```python
from build123d import *

# Parameters (mm, degrees)
BOSS_EXTRUDE1_DEPTH = 3.175
FILLET1_R           = 0.5
CUT_EXTRUDE2_REACH  = 51.643
SKETCH3_R           = 0.9652
FILLET2_R           = 1.5


with BuildPart() as part:
    # Model → Boss-Extrude1 (new body)
    with BuildSketch(Plane.XY):
        with BuildLine():
            Line((14.682892141, 1.324956628), (14.682892141, -14.675043372))
            Line((14.682892141, -14.675043372), (20.7298505, -14.675043372))
            ThreePointArc((20.7298505, -14.675043372), (25.4798505, -19.425043372), (20.7298505, -24.175043372))
            Line((20.7298505, -24.175043372), (11.5, -24.175043372))
            Line((11.5, -24.175043372), (11.5, -28.004155183))
            ThreePointArc((11.5, -28.004155183), (0.71022918, -27.624612518), (-8.091185045, -21.371748005))
            ThreePointArc((-8.091185045, -21.371748005), (-8.108719309, -19.937278968), (-6.731529764, -19.535585272))
            ThreePointArc((-6.731529764, -19.535585272), (3.21430247, -21.04378196), (8.674974651, -12.595391853))
            ThreePointArc((8.674974651, -12.595391853), (8.175614462, -12.09535774), (7.674976202, -12.594112234))
            ThreePointArc((7.674976202, -12.594112234), (3.234931854, -19.534945465), (-4.933394903, -18.4543911))
            Line((-4.933394903, -18.4543911), (-7.231528234, -16.526028271))
            ThreePointArc((-7.231528234, -16.526028271), (-5.055570769, -14.381233606), (-2.061467679, -14.989741395))
            ThreePointArc((-2.061467679, -14.989741395), (1.32956104, -15.458208706), (3.175, -12.575000001))
            Line((3.175, -12.575000001), (3.175, 12.575000001))
            ThreePointArc((3.175, 12.575000001), (-0.276719482, 15.737918167), (-3.126764616, 12.023667038))
            ThreePointArc((-3.126764616, 12.023667038), (-4.027590212, 8.661740144), (-7.182015159, 7.190807634))
            Line((-7.182015159, 7.190807634), (-38.940555286, 7.190807634))
            ThreePointArc((-38.940555286, 7.190807634), (-40.001215458, 7.630147462), (-40.440555286, 8.690807634))
            Line((-40.440555286, 8.690807634), (-40.440555286, 9.332781994))
            ThreePointArc((-40.440555286, 9.332781994), (-40.26291966, 10.040844464), (-39.772085337, 10.581204108))
            ThreePointArc((-39.772085337, 10.581204108), (-21.582497329, 19.5655863), (-1.704175076, 23.619293202))
            ThreePointArc((-1.704175076, 23.619293202), (14.213621823, 22.738093196), (29.39280733, 17.865198893))
            Line((29.39280733, 17.865198893), (29.39280733, 15.324956628))
            Line((29.39280733, 15.324956628), (11.5, 15.324956628))
            Line((11.5, 15.324956628), (11.5, 10.824956628))
            Line((11.5, 10.824956628), (20.7298505, 10.824956628))
            ThreePointArc((20.7298505, 10.824956628), (25.4798505, 6.074956628), (20.7298505, 1.324956628))
            Line((20.7298505, 1.324956628), (14.682892141, 1.324956628))
        make_face()
    extrude(amount=BOSS_EXTRUDE1_DEPTH)

    # Fillet1
    fillet1_edges = [part.edges().sort_by_distance(p)[0] for p in [
        (11.5, 15.324956628, 1.5875),
        (11.5, 10.824956628, 1.5875),
        (14.682892141, 1.324956628, 1.5875),
        (14.682892141, -14.675043372, 1.5875),
        (11.5, -24.175043372, 1.5875),
        (-7.231528234, -16.526028271, 1.5875),
    ]]
    fillet(fillet1_edges, radius=FILLET1_R)

    # Sketch3 → Cut-Extrude2 (cut, up to next)
    with BuildSketch(Plane(origin=(0, 0, 0), x_dir=(-1, 0, 0), z_dir=(0, 0, -1)), mode=Mode.PRIVATE) as cut_extrude2_sk1:
        with Locations((-20.7298505, 6.074956628)):
            Circle(SKETCH3_R)
    cut_extrude2_tool1 = extrude(cut_extrude2_sk1.sketch, amount=-CUT_EXTRUDE2_REACH, mode=Mode.PRIVATE) & part.part
    # Sketch3 → Cut-Extrude2 (cut, up to next)
    with BuildSketch(Plane(origin=(0, 0, 0), x_dir=(-1, 0, 0), z_dir=(0, 0, -1)), mode=Mode.PRIVATE) as cut_extrude2_sk2:
        with Locations((-20.7298505, -19.425043372)):
            Circle(SKETCH3_R)
    cut_extrude2_tool2 = extrude(cut_extrude2_sk2.sketch, amount=-CUT_EXTRUDE2_REACH, mode=Mode.PRIVATE) & part.part
    add(cut_extrude2_tool1.solids().sort_by_distance((20.729851, 6.074957, 0))[0], mode=Mode.SUBTRACT)
    add(cut_extrude2_tool2.solids().sort_by_distance((20.729851, -19.425043, 0))[0], mode=Mode.SUBTRACT)

    # Fillet2
    fillet2_edges = [part.edges().sort_by_distance(p)[0] for p in [
        (29.39280733, 17.865198893, 1.5875),
        (29.39280733, 15.324956628, 1.5875),
        (11.5, -28.004155183, 1.5875),
    ]]
    fillet(fillet2_edges, radius=FILLET2_R)


solid = part.part
```
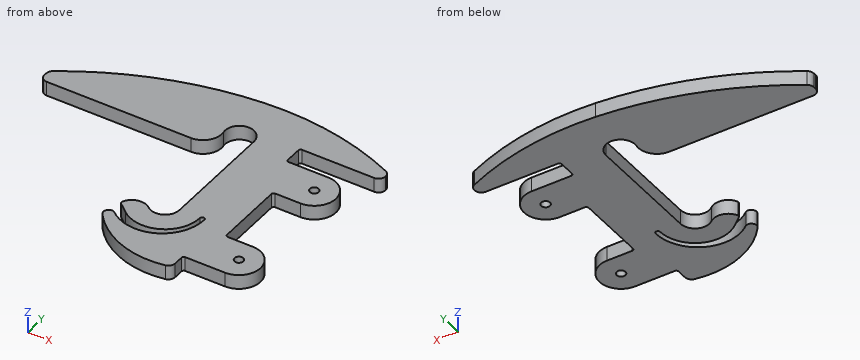
Model file for the job. Use its own axes, mm. Coordinates: 2 decimals unless noted, no trailing zeros. Write each loop counter-clockwise with the first axis right and the second up, starting at its lowest first coordinate (ties: lowest second). Pieces come first, ordered by that corner, then holes. Notation, with made-up numbers: (85.25, -30.75) - (92.25, -30.75) arc R18 cw to (92.25, -1.75) - close; hole circle Ø11 at (8.25, 42). An arc over 180 degrees is marked (long way). Use a Markdown table: item, result. Add a question column.
Item 1: Band-saw the part on B-B, the plane y = -5.5. Write the cut outline in (x, z) (3 decimals), and give its area (3 significant figures).
Item 2: Drop flat-ended pins along their axis: pin 1 (1.5 mm diameter, centred on x = 20.73, y = -19.43, fed in from -Z); pin 2 (1 mm diameter, centred on x = 19, z = 1.5, fed in from -Y); pin 3 (1.6 mm diameter, centred on x = 16.5, z = 2, fed in from +Y); pin 4 (1.7 mm diameter, centred on y = -26, z = 1, fed in from +X). Give the stop position or say it passes through.
Item 3: Band-saw the part on A-A, the plane x = 0. Give the number of separate pieces and of enclosed holes in the cut face, and give its area (3 significant figures).
Item 4: Band-saw the part on C-C, the plane x = 19. Write the cut outline in (y, z) (3 decimals), and give its area (3 significant figures).
Item 5: Drill centre lines: line 1 along Y through (x, z) = (0, 1.9); line 2 along X through (y, z) = (-20.5, 0.35); line 3 along Y through (x, z) = (2, 0.9). Where is each one in solid material? Low to high.
A:
| question | item | result |
|---|---|---|
| 1 | outline | (3.175, 0) - (14.683, 0) - (14.683, 3.175) - (3.175, 3.175) - close |
| 1 | area | 36.5 mm² |
| 2 | pin 1 | passes through |
| 2 | pin 2 | stops at y = -24.18 |
| 2 | pin 3 | stops at y = 22.44 |
| 2 | pin 4 | stops at x = 11.5 |
| 3 | separate pieces | 3 |
| 3 | enclosed holes | 0 |
| 3 | area | 57.1 mm² |
| 4 | outline | (-24.175, 0) - (-14.675, 0) - (-14.675, 3.175) - (-24.175, 3.175) - close; (1.325, 0) - (10.825, 0) - (10.825, 3.175) - (1.325, 3.175) - close; (15.325, 0) - (21.657, 0) - (21.657, 3.175) - (15.325, 3.175) - close |
| 4 | area | 80.4 mm² |
| 5 | line 1 | y = -27.37 to -21.84, -20.25 to -15.75, 15.75 to 23.72 |
| 5 | line 2 | x = -8.33 to -5.43, 4.24 to 25.36 |
| 5 | line 3 | y = -28.01 to -21.49, -19.98 to -15.04, 15.04 to 23.78 |
